Autodesk Inventor part; units mm, degrees
ref_plane "YZ Plane" through (0, 0, 0) normal (1, 0, 0) x (0, 1, 0)
ref_plane "XZ Plane" through (0, 0, 0) normal (0, 1, 0) x (-1, 0, 0)
ref_plane "XY Plane" through (0, 0, 0) normal (0, 0, 1) x (1, 0, 0)
sketch "Sketch1" plane through (0, 0, 0) normal (0, 1, 0) x (-1, 0, 0)
  line L0 (28, -85) -> (-28, -85)
  line L1 (-28, -85) -> (-28, 0)
  line L2 (-28, 0) -> (28, 0)
  line L3 (28, 0) -> (28, -85)
  point P0 (0, 0)
  point P1 (0, 0)
  dimension "d0" = 85
  dimension "d1" = 56
extrude "Extrusion1" add sketch "Sketch1" along normal blind 1.4
fillet "Fillet1" radius 3 4 edges at (-28, 0.7, 0) (28, 0.7, 0) (28, 0.7, -85) (-28, 0.7, -85)
sketch "Sketch2" plane through (0, 1.4, 0) normal (0, 1, 0) x (1, 0, 0)
  line L0 (-24.5, 61.5) -> (24.5, 61.5) construction
  line L1 (24.5, 61.5) -> (24.5, 3.5) construction
  line L2 (24.5, 3.5) -> (-24.5, 3.5) construction
  line L3 (-24.5, 3.5) -> (-24.5, 61.5) construction
  line L4 (-28, 82) -> (-28, 3) construction
  line L5 (-25, 0) -> (25, 0) construction
  point P0 (0, 0)
  dimension "d5" = 49
  dimension "d6" = 58
  dimension "d7" = 3.5
  dimension "d8" = 3.5
hole "Hole1" at (-24.5, 1.4, -61.5) at (24.5, 1.4, -61.5) at (24.5, 1.4, -3.5) at (-24.5, 1.4, -3.5) direction (0, -1, 0) diameter 3 depth 6
properties part number "raspberry pi"
Can you work these out from the model? Positions are in its coordinate system, mm. Round coordinates to 2 decimals unless told otherwise and drop trailing zeros. Order: outer loops, then holes, each group sorted by start corner. A loop starts at its lowest first (then second) coordinate and runs counter-clockwise, first axis right, second up.
(1) If we section it at A-A (z = -61.5): Please give me the cut outline in (x, y), plus the area to 3 significant figures.
Results are:
outline: (-28, 0) - (-26, 0) - (-26, 1.4) - (-28, 1.4) - close; (-23, 0) - (23, 0) - (23, 1.4) - (-23, 1.4) - close; (26, 0) - (28, 0) - (28, 1.4) - (26, 1.4) - close
area: 70.0 mm2
(2) We'd pull the mould along Z, two halves only. Please class faces 1 (the face through (23.013, 0.69, -3.695)), 2 (the face through (-27.1, 0.71, -84.14)), 3 (the face through (-25.987, 0.69, -3.695)), 4 (the face through (0, 0, -42)): +Z half, -Z half, draft (parallel to the pull), parting line (faces both ways), or undercut.
Results are:
face 1: undercut
face 2: -Z half
face 3: undercut
face 4: draft
(3) If I drill on L1, parallel to Z at x = -24.5, y = 0.6; L2, parallel to X at y = 0.7, z = -61.5; L3, parallel to Z at x = -24, y = 0.3, over which ranges is the centre line in solid material (lowest first)?
Results are:
L1: z = -85 to -63, -60 to -5, -2 to 0
L2: x = -28 to -26, -23 to 23, 26 to 28
L3: z = -85 to -62.91, -60.09 to -4.91, -2.09 to 0
